Could you check a few things on this model? Use its own coordinates, in mm. Face numbers are marked on the shaded views. Give positions to 0.01 mm unless a question says otherwise; leave off trailing zeros. Write each loop counter-clockwise with the first axis right and the second up, starting at its lowest first coordinate (ties: lowest second). Pieces come first, ordered by that corner, then holes. Notation, with made-up numbers: (-35, -31) - (-12, -31) arc R17 cw to (-12, -4) - close; hole circle Ø1 at (-26, -33). An arc over 180 degrees is marked (long way). Use one line per item in the form item = value.
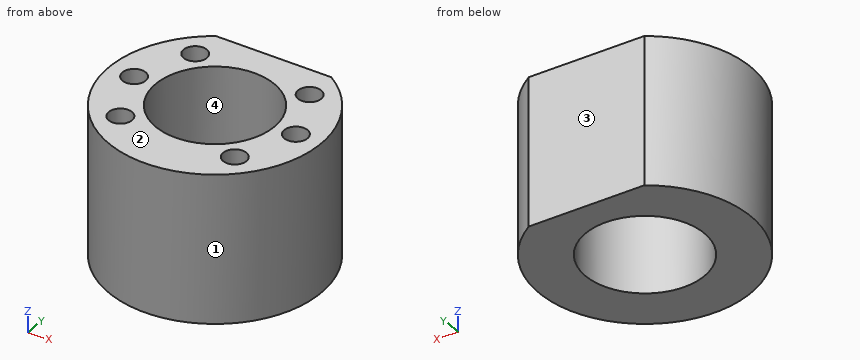
```python
from build123d import *

# Parameters (mm, degrees)
SKETCH1_R           = 25
SKETCH1_R_2         = 14
BOSS_EXTRUDE1_DEPTH = 35
CUT_EXTRUDE1_REACH  = 37
SKETCH2_W           = 99.603023316
SKETCH2_H           = 15.412230785
SKETCH3_R           = 2.75
CUT_EXTRUDE2_DEPTH  = 16


with BuildPart() as part:
    # Sketch1 → Boss-Extrude1 (new body)
    with BuildSketch(Plane.XY):
        Circle(SKETCH1_R)
        Circle(SKETCH1_R_2, mode=Mode.SUBTRACT)
    extrude(amount=BOSS_EXTRUDE1_DEPTH)

    # Sketch2 → Cut-Extrude1 (cut, up to next)
    with BuildSketch(Plane.XY.offset(35), mode=Mode.PRIVATE) as cut_extrude1_sk1:
        with Locations((-3.888962486, 28.706115393)):
            Rectangle(SKETCH2_W, SKETCH2_H)
    cut_extrude1_tool1 = extrude(cut_extrude1_sk1.sketch, amount=-CUT_EXTRUDE1_REACH, mode=Mode.PRIVATE) & part.part
    add(cut_extrude1_tool1.solids().sort_by_distance((-3.888962, 28.706115, 35))[0], mode=Mode.SUBTRACT)

    # Sketch3 → Cut-Extrude2 (cut)
    with BuildSketch(Plane.XY.offset(35)):
        with Locations((-13.435028843, 13.435028843)):
            Circle(SKETCH3_R)
        with Locations((-19, 0)):
            Circle(SKETCH3_R)
        with Locations((-13.435028843, -13.435028843)):
            Circle(SKETCH3_R)
    cut_extrude2 = extrude(amount=-CUT_EXTRUDE2_DEPTH, mode=Mode.SUBTRACT)

    # Mirror1: Cut-Extrude2 across plane
    add(cut_extrude2.mirror(Plane(origin=(0, 0, 0), x_dir=(0, 0, 1), z_dir=(1, 0, 0))), mode=Mode.SUBTRACT)


solid = part.part
```
1. Imagine slicing it at D-D, the plane z = 22. List the corners of the cut face in (x, y) for me.
Response values:
outline = (-13.56, 21) arc R25 ccw (long way) to (13.56, 21) - close; hole circle Ø5.5 at (-19, 0); hole circle Ø5.5 at (-13.44, -13.44); hole circle Ø5.5 at (-13.44, 13.44); hole circle Ø28 at (0, 0); hole circle Ø5.5 at (13.44, -13.44); hole circle Ø5.5 at (13.44, 13.44); hole circle Ø5.5 at (19, 0)
2. If I drill on line 1 (Y direction, x = 19, z = 25); line 2 (X direction, y = -14.5, z = 23); line 3 (X direction, y = 15, z = 24.5), over which ranges is the centre line in solid material (lowest first)? Write a range as from..to.
Response values:
line_1 = -16.25..-2.75, 2.75..16.25
line_2 = -20.37..-15.97, -10.9..10.9, 15.97..20.37
line_3 = -20..-15.7, -11.17..11.17, 15.7..20
3. Imagine slicing it at B-B, the plane x = -9. List the corners of the cut face in (y, z) for me, and give its area (3 significant figures).
Response values:
outline = (-23.32, 0) - (-10.72, 0) - (-10.72, 35) - (-23.32, 35) - close; (10.72, 0) - (21, 0) - (21, 35) - (10.72, 35) - close
area = 801 mm²
4. Imagine slicing it at A-A, the plane y = 0. List the corners of the cut face in (x, z) for me.
Response values:
outline = (-25, 0) - (-14, 0) - (-14, 35) - (-16.25, 35) - (-16.25, 19) - (-21.75, 19) - (-21.75, 35) - (-25, 35) - close; (14, 0) - (25, 0) - (25, 35) - (21.75, 35) - (21.75, 19) - (16.25, 19) - (16.25, 35) - (14, 35) - close
5. Imagine slicing it at C-C, the plane z = 3. List the corners of the cut face in (x, y) for me, and give its area (3 significant figures).
Response values:
outline = (-13.56, 21) arc R25 ccw (long way) to (13.56, 21) - close; hole circle Ø28 at (0, 0)
area = 1,270 mm²
6. For pin 1 (6.5 mm diameter, centred on x = 13.44, y = -13.44, fed in from -Z); pin 2 (10 mm diameter, centred on y = -7.5, z = 7, fed in from +X); pin 3 (8 mm diameter, centred on x = 5.5, y = -3.5, fed in from -Z); pin 4 (1.6 mm diameter, centred on x = -14.5, y = 13.5, fed in from +Z), each with a flat end and sliding along its axis, tell me the tip position at first contact or that it passes through.
Response values:
pin_1 = 0
pin_2 = 24.87
pin_3 = through
pin_4 = 19
7. If we mould it in two halves opening along Y, with no side actions, what happens to the marked faces 1, 2, 3 and 4? For each: pulls with the +Y half, pulls with the -Y half, needs draft (parallel to the pull), parting line crosses it, or undercut.
Response values:
face_1 = parting line crosses it
face_2 = needs draft
face_3 = pulls with the +Y half
face_4 = undercut
